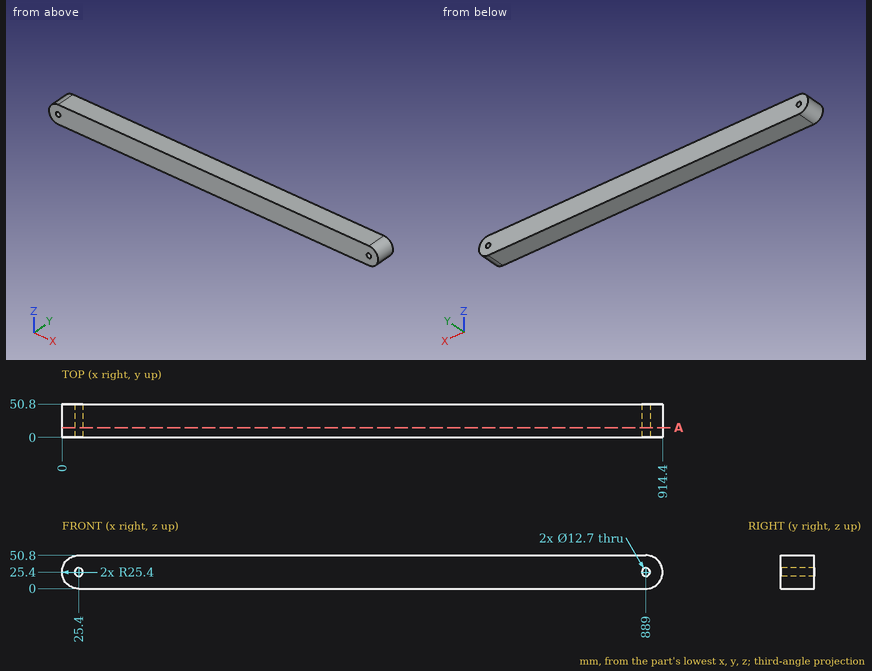
Design review of the part shown in the three views and the two pictorial views. Dimensions are in mm from the part's minimum x, y and z. Give positions to 0.01 mm unless a question says otherwise; leave off trailing zeros. Loops run counter-clockwise (first coordinate to the right, second up) from the corner with the lowest first, then second, coordinate; pieces in that order, holes last. Notation, with made-up numbers: M 70,70.25 L 102,70.25 A32 ccw 102,99.25 Z; hole C 16,5.5 d1. An arc over 180 degrees is marked long. Answer as a JSON object with one key per item and string values. Group by question number.
Q1. Add section A-A on y = 15. Give the boundary of the cut face in (x, z).
Q2. For probe 1 along X at (y, z) = (29, 24.5); probe 2 along Z at (x, y) = (889, 30); probe 3 along X at (y, z) = (45.5, 13), list the stretches that pass through material, from the lowest coordinate up. Write a range as [from, to].
Q3. Insertion check: P1, Ø10, axis at y = 32.5, z = 25.5, coming from the -X side; P2, Ø10, axis at x = 889, z = 25.4, coming from the -Y side; P3, Ø1.5, axis at y = 21.5, z = 20.5, coming from the -X side; P4, Ø5, axis at y = 28, z = 9, coming from the -X side. Each pin has a flat end and moves straight along its axis. Give the tip position at first contact, or say it passes through.
Checked values:
{
 "1": {"outline": "M 25.4,0 L 889,0 A25.4 ccw 889,50.8 L 25.4,50.8 A25.4 ccw Z; hole C 25.4,25.4 d12.7; hole C 889,25.4 d12.7"},
 "2": {"probe 1": "[0.02, 19.11], [31.69, 882.71], [895.29, 914.38]", "probe 2": "[0, 19.05], [31.75, 50.8]", "probe 3": "[3.23, 911.17]"},
 "3": {"P1": "x = 0", "P2": "through", "P3": "x = 0.34", "P4": "x = 4.14"}
}
